from build123d import *

# Parameters (mm, degrees)
ESBO_O1_W                    = 350
ESBO_O1_H                    = 205
RESSALTO_EXTRUS_O1_DEPTH     = 6
CORTE_EXTRUS_O1_DEPTH        = 203.897141429
FURO_DE_DI_METRO_4_2_4_2_1_D = 4.2


with BuildPart() as part:
    # Esboço1 → Ressalto-extrusão1 (new body)
    with BuildSketch(Plane.XY):
        Rectangle(ESBO_O1_W, ESBO_O1_H)
    extrude(amount=RESSALTO_EXTRUS_O1_DEPTH)

    # Esboço2 → Corte-extrusão1 (cut, through all)
    with BuildSketch(Plane.XY.offset(6)):
        with BuildLine():
            Line((-37.5, 60), (37.5, 60))
            ThreePointArc((37.5, 60), (47.5, 50), (37.5, 40))
            Line((37.5, 40), (-37.5, 40))
            ThreePointArc((-37.5, 40), (-47.5, 50), (-37.5, 60))
        make_face()
    extrude(amount=-CORTE_EXTRUS_O1_DEPTH, mode=Mode.SUBTRACT)

    # Furo de diâmetro Ø4.2 (4.2)1 (through all)
    with Locations(Plane(origin=(0, 0, 0), x_dir=(-1, 0, 0), z_dir=(0, 0, -1))):
        with Locations((-151, -87.5), (-151, -18), (-151, 28.5), (-151, 78), (151, -77.5), (151, -28), (151, 18.5), (151, 88)):
            Hole(FURO_DE_DI_METRO_4_2_4_2_1_D / 2)


solid = part.part
Work out the finished part from the listing and answer in its coordinate system (mm). A direction names the side the tool comes from. Give positions to 0.01 mm unless a question says otherwise; leave off trailing zeros. Loops run counter-clockwise (first coordinate to the right, second up) from the corner with the lowest first, then second, coordinate; pieces in that order, holes last. Notation, with made-up numbers: M 72,41.25 L 108,41.25 A28 ccw 108,75.25 Z; hole C 0,44 d4. An arc over 180 degrees is marked long. Use CSV: the item, a comma, the result in double quotes.
1) Given P1, Ø4, axis at x = -151, y = -77.5, coming from the -Z side; P2, Ø5, axis at x = -151, y = 18.5, coming from the -Z side, each flat-ended and moving along its own axis, determine where each tip first touches the part or whether it passes through.
Answer:
P1,"through"
P2,"z = 0"
2) Consider L1, parallel to Y at x = -151, z = 2.65; L2, parallel to Y at x = 151, z = 4.15; L3, parallel to Y at x = 10.5, z = 5.15. Determine where each line is inside the solid, lowest interval first.
Answer:
L1,"-102.5 to -79.6, -75.4 to -30.1, -25.9 to 16.4, 20.6 to 85.9, 90.1 to 102.5"
L2,"-102.5 to -89.6, -85.4 to -20.1, -15.9 to 26.4, 30.6 to 75.9, 80.1 to 102.5"
L3,"-102.5 to 40, 60 to 102.5"
3) Find section B-B on y = 47.5. Write down the section's boundary in (x, z), plus the area to 3 significant figures.
Answer:
outline,"M -175,0 L -47.18,0 L -47.18,6 L -175,6 Z; M 47.18,0 L 175,0 L 175,6 L 47.18,6 Z"
area,"1,530 mm^2"
4) Find section A-A on z = 5.1. Give the number of separate pieces and of enclosed holes in the cut face, plus the area to 3 significant figures.
Answer:
separate pieces,"1"
enclosed holes,"9"
area,"69,800 mm^2"
5) Which of the six approach directions +Z, -Z, +X, -X, +Y, -Y give full straight-line access (tool end or side, diameter ignored) to faces 1 (the cylindrical face through (-47.5, 49.8, 3)), 2 (the flat face through (-2, 1, 0))?
Answer:
face 1,"+Z, -Z"
face 2,"-Z, +X, -X, +Y, -Y"
